from build123d import *

# Parameters (mm, degrees)
SKETCH_R     = 2
PAD_DEPTH    = 14
POCKET_DEPTH = 5


with BuildPart() as part:
    # Sketch → Pad (new body)
    with BuildSketch(Plane.XY):
        with BuildLine():
            Line((-16, 18), (7, 18))
            ThreePointArc((8, 17), (7.707107, 17.707107), (7, 18))
            Line((8, 17), (8, 11))
            ThreePointArc((7, 10), (7.707107, 10.292893), (8, 11))
            Line((7, 10), (0, 10))
            Line((0, 10), (0, 0))
            Line((0, 0), (-23, 0))
            ThreePointArc((-24, 1), (-23.707107, 0.292893), (-23, 0))
            Line((-24, 1), (-24, 7))
            ThreePointArc((-23, 8), (-23.707107, 7.707107), (-24, 7))
            Line((-23, 8), (-16, 8))
            Line((-16, 8), (-16, 18))
        make_face()
        with Locations((4, 14)):
            Circle(SKETCH_R, mode=Mode.SUBTRACT)
        with Locations((-20, 4)):
            Circle(SKETCH_R, mode=Mode.SUBTRACT)
    extrude(amount=PAD_DEPTH)

    # Sketch001 → Pocket (cut)
    with BuildSketch(Plane.XY):
        Polygon((-2.35, 18), (-2.35, 0), (-10.75, 0), (-14.35, 18), align=None)
    extrude(amount=POCKET_DEPTH, mode=Mode.SUBTRACT)


solid = part.part
For this review, take the finished solid that the model builds, in its own axes (mm). A direction names the side the tool comes from. Give positions to 0.01 mm unless a question says otherwise; leave off trailing zeros. Write each loop counter-clockwise with the first axis right and the second up, starting at its lowest first coordinate (ties: lowest second). Pieces come first, ordered by that corner, then holes. Notation, with made-up numbers: (56.5, 74.5) -> (62.5, 74.5) arc R15 ccw to (62.5, 86.5) -> close; hole circle Ø7 at (8, 9.25). An arc over 180 degrees is marked (long way). Use CSV: the item, a comma, the result in double quotes.
Q1. To check wall thickness, follow probe 1 along Y at (x, z) = (-20, 9.5); probe 2 along Y at (x, z) = (4, 4); probe 3 along X at (y, z) = (8.75, 6). State the ranges of each line that lie inside material, in increasing order. Write a range as [from, to].
Conclusion:
probe 1,"[0, 2], [6, 8]"
probe 2,"[10, 12], [16, 18]"
probe 3,"[-16, 0]"
Q2. Take a section at B-B, the plane y = 14. Write out the cut boundary in (x, z).
Conclusion:
outline,"(-16, 0) -> (-13.55, 0) -> (-13.55, 5) -> (-2.35, 5) -> (-2.35, 0) -> (2, 0) -> (2, 14) -> (-16, 14) -> close; (6, 0) -> (8, 0) -> (8, 14) -> (6, 14) -> close"
Q3. Take a section at A-A, the plane x = 4. Write out the cut boundary in (y, z).
Conclusion:
outline,"(10, 0) -> (12, 0) -> (12, 14) -> (10, 14) -> close; (16, 0) -> (18, 0) -> (18, 14) -> (16, 14) -> close"
Q4. Mouldability with a two-part tool opening along X and no side actions: class faces 6 (the face through (-8, 9, 14)), 7 (the face through (-21.6, 2.8, 6.9)), 8 (the face through (7.715, 17.699, 6.902)), 9 (the face through (-16, 13, 7)) as pulls with the +X half, pulls with the -X half, needs draft (parallel to the pull), parting line crosses it, or undercut.
Conclusion:
face 6,"needs draft"
face 7,"undercut"
face 8,"pulls with the +X half"
face 9,"pulls with the -X half"
Q5. Take a section at C-C, the plane z = 2.25. Write out the cut boundary in (x, y).
Conclusion:
outline,"(-24, 1) arc R1 ccw to (-23, 0) -> (-10.75, 0) -> (-14.35, 18) -> (-16, 18) -> (-16, 8) -> (-23, 8) arc R1 ccw to (-24, 7) -> close; (-2.35, 0) -> (0, 0) -> (0, 10) -> (7, 10) arc R1 ccw to (8, 11) -> (8, 17) arc R1 ccw to (7, 18) -> (-2.35, 18) -> close; hole circle Ø4 at (-20, 4); hole circle Ø4 at (4, 14)"
Q6. Tool access review of faces 1 (the face through (-20, 8, 7)), 2 (the face through (-12.525, 8.874, 2.465)), 3 (the face through (0, 5, 7)), 4 (the face through (-24, 4, 7)), 5 (the face through (-2.35, 9, 2)): name each direction out of +Z, -Z, +X, -X, +Y, -Y from which nothing blocks a thin tool from reaching the whole face with its end or side.
Conclusion:
face 1,"+Z, -Z, -X, +Y"
face 2,"-Z, +Y"
face 3,"+Z, -Z, +X, -Y"
face 4,"+Z, -Z, -X, +Y, -Y"
face 5,"-Z, +Y, -Y"
Q7. Take a section at D-D, the plane y = 6.5. Write out the cut boundary in (x, z), then the cut area to 4 significant figures.
Conclusion:
outline,"(-24, 0) -> (-12.05, 0) -> (-12.05, 5) -> (-2.35, 5) -> (-2.35, 0) -> (0, 0) -> (0, 14) -> (-24, 14) -> close"
area,"287.5 mm2"
Q8. For P1, Ø3.5, axis at x = -21, z = 6.5, coming from the +Y side; P2, Ø2, axis at x = 4, z = 5, coming from the -Y side; P3, Ø5, axis at y = 3.5, z = 4.5, coming from the +X side, all flat-tipped, find the tip position at first contact; note any pin that passes through.
Conclusion:
P1,"y = 8"
P2,"y = 10"
P3,"x = 0"
